Source: three-view drawing plus pictorial views. Frame: mm from the lowest corner of the part. Give positions to 0.01 mm unless a question says otherwise; leave off trailing zeros. Loops run counter-clockwise (first coordinate to the right, second up) from the corner with the lowest first, then second, coordinate; pieces in that order, holes last. Notation, with made-up numbers: (-32.75, 14.25) -> (5.25, 14.25) arc R22 cw to (5.25, 34.25) -> close; hole circle Ø7 at (24, 2.5). An arc over 180 degrees is marked (long way). One line per item, written item: value. Start each with the question number.
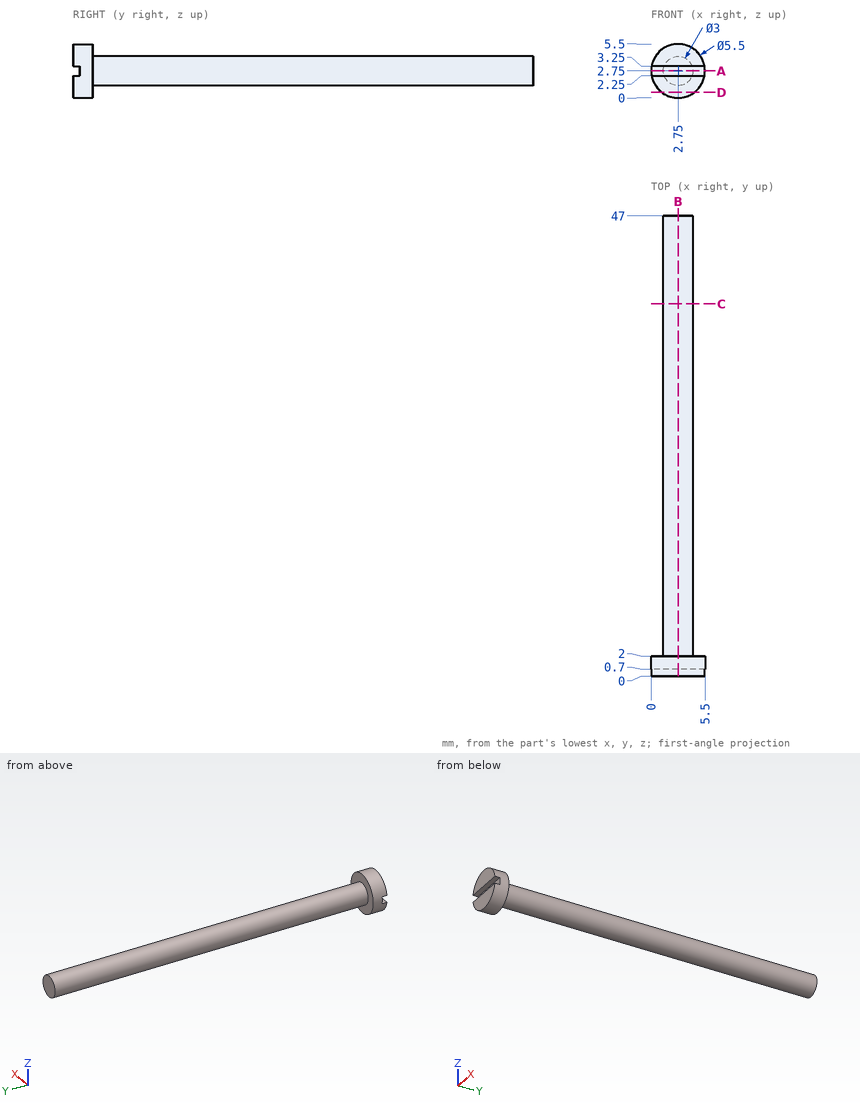
Item 1: Pin query (flat end, axial travel): pin 1 (0.6 mm diameter, centred on x = 3.5, y = 0.5, fed in from +Z); pin 2 (2 mm diameter, centred on y = 38, z = 2, fed in from +X); pin 3 (3 mm diameter, centred on x = 4, y = 32.5, fed in from +Z). Return the tip coordinate at first contact, or that it passes through.
Item 2: Section C-C, the plane y = 38. Output: boundary loops of the cut face in (x, z), then the cut area to 3 significant figures.
Item 3: Ray query, line 1 along Y through (x, z) = (3.3, 4.55); line 2 along Y through (x, z) = (5.05, 2.6); line 3 along X through (y, z) = (36, 2.7). Return the intervals inside material, ascending. Write a range as [from, to].
Item 4: Section B-B, the plane x = 2.75. Output: boundary loops of the cut face in (y, z).
Item 5: Section A-A, the plane z = 2.75. Output: boundary loops of the cut face in (x, y).
Item 6: Section D-D, the plane z = 0.55. Output: boundary loops of the cut face in (x, y).
Geometry check:
1. pin 1: stops at z = 5.46
1. pin 2: stops at x = 4.25
1. pin 3: stops at z = 4.25
2. outline: circle Ø3 at (2.75, 2.75)
2. area: 7.07 mm2
3. line 1: y = [0, 2]
3. line 2: y = [0.7, 2]
3. line 3: x = [1.25, 4.25]
4. outline: (0, 0) -> (2, 0) -> (2, 1.25) -> (47, 1.25) -> (47, 4.25) -> (2, 4.25) -> (2, 5.5) -> (0, 5.5) -> (0, 3.25) -> (0.7, 3.25) -> (0.7, 2.25) -> (0, 2.25) -> close
5. outline: (0, 0.7) -> (5.5, 0.7) -> (5.5, 2) -> (4.25, 2) -> (4.25, 47) -> (1.25, 47) -> (1.25, 2) -> (0, 2) -> close
6. outline: (1.1, 0) -> (4.4, 0) -> (4.4, 2) -> (1.1, 2) -> close
